The drawing under review shows one solid part. Ordinate dimensions are in mm from its lowest x, y, z. Round coordinates to 2 decimals unless told otherwise and drop trailing zeros. Write each loop counter-clockwise with the first axis right and the second up, starting at its lowest first coordinate (ties: lowest second). Pieces come first, ordered by that corner, then holes. Notation, with made-up numbers: (64.25, 63.5) -> (110.25, 63.5) arc R8 cw to (110.25, 72.5) -> close; hole circle Ø7 at (77, 34.5). An arc over 180 degrees is marked (long way). Write item = value, one per line. Start each with the question number.
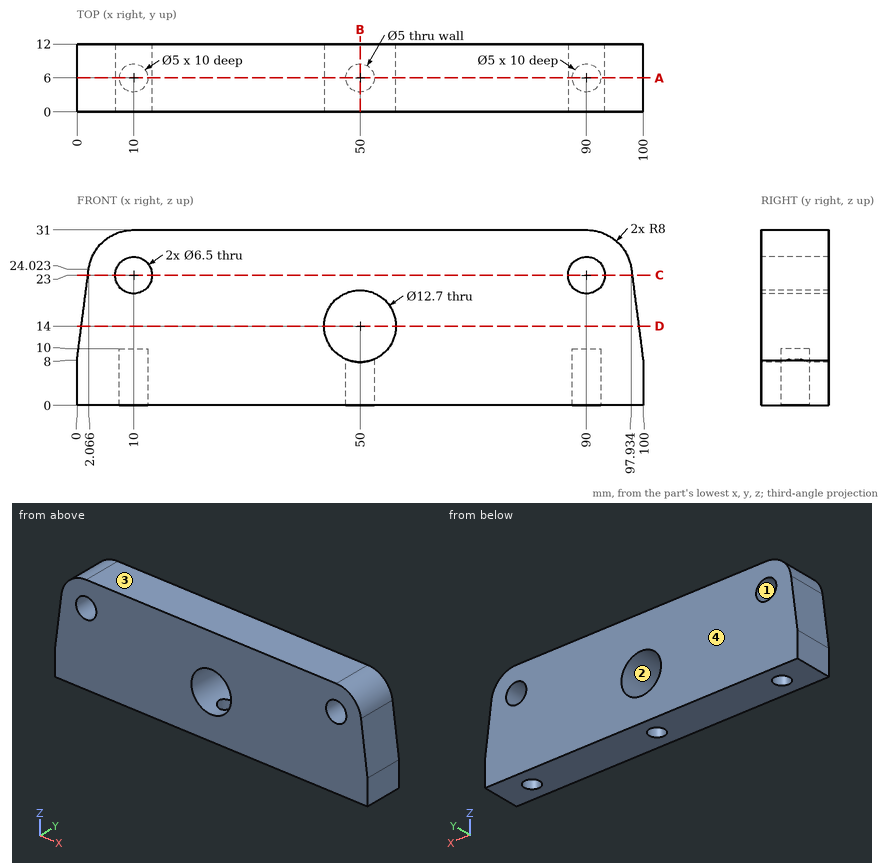
1. Consider section A-A, the plane y = 6. Give the number of separate pieces and of enclosed holes in the cut face, then the cut area to 3 significant figures.
2. Consider section C-C, the plane z = 23. Give the boundary of the cut face in (x, y).
3. Clearance check with flat-ended pins moving along their axes: pin 1 Ø16.5 at (x, z) = (50, 14) entering from -Y; pin 2 Ø4 at (x, y) = (50, 6) entering from -Z; pin 3 Ø4 at (y, z) = (4, 11.5) entering from -X; pin 4 Ø3 at (x, y) = (10, 6) entering from -Z. State where each tip first meets the part, or that it passes through.
4. Wall thickness on L1, parallel to Z at x = 10, y = 5.5; L2, parallel to Z at x = 10, y = 9.5; L3, parallel to X at y = 7.5, z = 25.5 (1 decimal): over which ranges is each line inside the solid? List them lowest first. Write a range as from..to.
5. Draft analysis for pull direction Z (two halves, no side actions). For the marked faces 1, 2, 3 and 4, state which applies: +Z half, -Z half, draft (parallel to the pull), parting line (faces both ways), or undercut.
6. Consider section B-B, the plane x = 50. Give the boundary of the cut face in (y, z).
7. Consider section D-D, the plane z = 14. Give the boundary of the cut face in (x, y).
Outcome:
q1.separate_pieces = 1
q1.enclosed_holes = 2
q1.area = 2,680 mm2
q2.outline = (1.93, 0) -> (6.75, 0) -> (6.75, 12) -> (1.93, 12) -> close; (13.25, 0) -> (86.75, 0) -> (86.75, 12) -> (13.25, 12) -> close; (93.25, 0) -> (98.07, 0) -> (98.07, 12) -> (93.25, 12) -> close
q3.pin_1 = 0
q3.pin_2 = 20.03
q3.pin_3 = 0.19
q3.pin_4 = 10
q4.L1 = 10..19.75, 26.25..31
q4.L2 = 0..19.75, 26.25..31
q4.L3 = 2.4..7.9, 12.1..87.9, 92.1..97.6
q5.face_1 = undercut
q5.face_2 = undercut
q5.face_3 = +Z half
q5.face_4 = draft
q6.outline = (0, 0) -> (3.5, 0) -> (3.5, 7.65) -> (0, 7.65) -> close; (0, 20.35) -> (12, 20.35) -> (12, 31) -> (0, 31) -> close; (8.5, 0) -> (12, 0) -> (12, 7.65) -> (8.5, 7.65) -> close
q7.outline = (0.77, 0) -> (43.65, 0) -> (43.65, 12) -> (0.77, 12) -> close; (56.35, 0) -> (99.23, 0) -> (99.23, 12) -> (56.35, 12) -> close
